For this review, take the finished solid that the model builds, in its own axes (mm). A direction names the side the tool comes from. Round coordinates to 2 decimals unless told otherwise and drop trailing zeros. Loops run counter-clockwise (first coordinate to the right, second up) from the corner with the lowest first, then second, coordinate; pieces in that order, holes last.
1. To check wall thickness, follow line 1 along Y through (x, z) = (0, 18.95); line 2 along Z through (x, y) = (-16, 9); line 3 along Y through (x, z) = (-5.5, 6). State the ranges of each line that lie inside material, in increasing order.
2. Consider section A-A on x = 0. State the section outline as (y, z) points.
3. Tool access review of faces 1 (the cylindrical face through (14.985, 0.66, 7.888)), 2 (the flat face through (3, 15, 16)): name each direction out of +Z, -Z, +X, -X, +Y, -Y from which nothing blocks a thin tool from reaching the whole face with its end or side.
4. Draft analysis for pull direction X (two halves, no side actions). For faces 3 (the flat face through (6, 14, 0)), 4 (the conical face through (-6.12, -27.54, 14.58)), 5 (the cylindrical face through (-4.336, -19.524, 18.028)), state which applies: released by +X, released by -X, zero draft, split by the parting line, or undercut.
5. Clearance check with flat-ended pins moving along their axes: pin 1 Ø1.5 at (y, z) = (-23.5, 11) entering from -X; pin 2 Ø3 at (x, y) = (9, -13.5) entering from -Z; pin 3 Ø3 at (y, z) = (-12.5, 3.5) entering from -X; pin 4 Ø1 at (y, z) = (-6.5, 5.5) entering from -X. State where each tip first meets the part, or that it passes through.
6. Consider section C-C on z = 10. State the section outline as (x, y) points.
7. Consider section D-D on z = 14.75. State the section outline as (x, y) points.
from build123d import *

# Parameters (mm, degrees)
SKETCH1_R           = 30
BOSS_EXTRUDE1_DEPTH = 20
BOSS_EXTRUDE1_TAPER = 7
SKETCH3_R           = 15
CUT_EXTRUDE1_DEPTH  = 21
SKETCH5_R           = 20
CUT_EXTRUDE2_DEPTH  = 4


with BuildPart() as part:
    # Sketch1 → Boss-Extrude1 (new body)
    with BuildSketch(Plane.XY):
        Circle(SKETCH1_R)
    extrude(amount=BOSS_EXTRUDE1_DEPTH, taper=BOSS_EXTRUDE1_TAPER)

    # Sketch3 → Cut-Extrude1 (cut, through all)
    with BuildSketch(Plane(origin=(0, 0, 0), x_dir=(-1, 0, 0), z_dir=(0, 0, -1))):
        Circle(SKETCH3_R)
    extrude(amount=-CUT_EXTRUDE1_DEPTH, mode=Mode.SUBTRACT)

    # Sketch5 → Cut-Extrude2 (cut)
    with BuildSketch(Plane.XY.offset(20)):
        Circle(SKETCH5_R)
    extrude(amount=-CUT_EXTRUDE2_DEPTH, mode=Mode.SUBTRACT)


solid = part.part
Resolved:
1. line 1: y = -27.67 to -20, 20 to 27.67
1. line 2: z = 0 to 16
1. line 3: y = -28.74 to -13.96, 13.96 to 28.74
2. outline: (-30, 0) - (-15, 0) - (-15, 16) - (-20, 16) - (-20, 20) - (-27.54, 20) - close; (15, 0) - (30, 0) - (27.54, 20) - (20, 20) - (20, 16) - (15, 16) - close
3. face 1: +Z, -Z
3. face 2: +Z
4. face 3: zero draft
4. face 4: split by the parting line
4. face 5: undercut
5. pin 1: stops at x = -17.42
5. pin 2: stops at z = 0
5. pin 3: stops at x = -27.48
5. pin 4: stops at x = -28.72
6. outline: circle Ø57.54 at (0, 0); hole circle Ø30 at (0, 0)
7. outline: circle Ø56.38 at (0, 0); hole circle Ø30 at (0, 0)
